The drawing under review shows one solid part. Ordinate dimensions are in mm from its lowest x, y, z. A direction names the side the tool comes from. Give positions to 0.01 mm unless a question says otherwise; leave off trailing zeros. Loops run counter-clockwise (first coordinate to the right, second up) from the corner with the lowest first, then second, coordinate; pieces in that order, holes last. Notation, with made-up numbers: M -22,-14.5 L 35,-14.5 A16 cw 35,-6.5 Z; hole C -23.75,20 d11. An arc over 180 degrees is marked long. Answer as CSV lines item,"result".
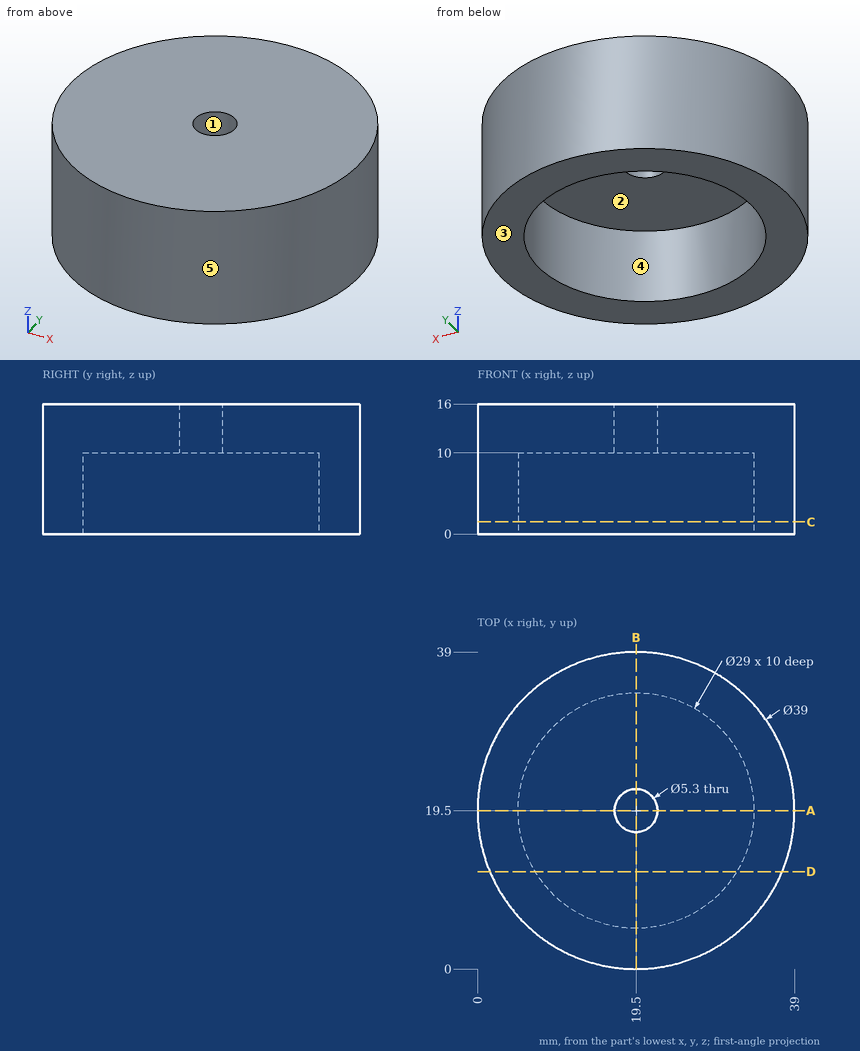
1. To check wall thickness, follow L1, parallel to Y at x = 19.5, z = 12.5; L2, parallel to Z at x = 14, y = 20.5; L3, parallel to X at y = 22, z = 2.5. State the ranges of each line that lie inside material, in increasing order. Write a range as [from, to].
Answer block:
L1,"[0, 16.85], [22.15, 39]"
L2,"[10, 16]"
L3,"[0.16, 5.22], [33.78, 38.84]"
2. We need section D-D, the plane y = 12. Write out the cut boundary in (x, z), plus the area to 3 significant figures.
Answer block:
outline,"M 1.5,0 L 7.09,0 L 7.09,10 L 31.91,10 L 31.91,0 L 37.5,0 L 37.5,16 L 1.5,16 Z"
area,"328 mm²"
3. We need section C-C, the plane z = 1.5. Write out the cut boundary in (x, y).
Answer block:
outline,"C 19.5,19.5 d39; hole C 19.5,19.5 d29"
4. We need section A-A, the plane y = 19.5. Write out the cut boundary in (x, z), plus the area to 3 significant figures.
Answer block:
outline,"M 0,0 L 5,0 L 5,10 L 16.85,10 L 16.85,16 L 0,16 Z; M 22.15,10 L 34,10 L 34,0 L 39,0 L 39,16 L 22.15,16 Z"
area,"302 mm²"
5. For P1, Ø8.5, axis at x = 24, y = 24.5, coming from the -Z side; P2, Ø5, axis at x = 19.5, y = 19.5, coming from the +Z side; P3, Ø4, axis at x = 30, z = 11, coming from the -Y side; P4, Ø1.5, axis at x = 24.5, z = 11.5, coming from the -Y side, all flat-tipped, find the tip position at first contact; note any pin that passes through.
Answer block:
P1,"z = 10"
P2,"through"
P3,"y = 1.95"
P4,"y = 0.47"
6. For the marked faces 1 and 2, list the 3-axis set-ups (+Z, -Z, +X, -X, +Y, -Y) from which the entire face can be reached by the end or side of a thin tool; tool diameter is ignored.
Answer block:
face 1,"+Z, -Z"
face 2,"-Z"
7. The part is to be moulded in two halves that separate along X. For the marked faces 3, 4 and 5, say which applies: pulls with the +X half, pulls with the -X half, needs draft (parallel to the pull), parting line crosses it, or undercut.
Answer block:
face 3,"needs draft"
face 4,"undercut"
face 5,"parting line crosses it"
